Work out the finished part from the listing and answer in its coordinate system (mm). A direction names the side the tool comes from. Coordinates: 2 decimals unless noted, no trailing zeros. Loops run counter-clockwise (first coordinate to the right, second up) from the corner with the lowest first, then second, coordinate; pieces in that order, holes last. Notation, with made-up numbers: (43.25, 26.5) - (51.25, 26.5) arc R9 cw to (51.25, 42.5) - close; hole circle Ø7 at (80, 82). An arc over 180 degrees is marked (long way). Write each question's results on one line, items separated by ' | '. Start each with the question number.
Item 1: Section A-A, the plane x = -9.75 is taken. Write down the section's boundary in (y, z), plus the area to 3 significant figures.
Item 2: Section C-C, the plane y = 6.75 is taken. Write down the section's boundary in (x, z), plus the area to 3 significant figures.
Item 3: Section B-B, the plane x = 0 is taken. Write down the section's boundary in (y, z) (3 decimals).
Item 4: Each of these flat-tipped pins is pushed along its axis until it touches: pin 1 Ø2.5 at (y, z) = (-4.5, -0.5) entering from -X; pin 2 Ø3 at (x, y) = (2, 9) entering from -Z; pin 3 Ø10 at (x, y) = (6.5, 6) entering from -Z; pin 4 Ø0.6 at (y, z) = (-2, -1.5) entering from +X (3 decimals). Where does it stop, or does it pass through?
Item 5: A tool of negligible diameter and unlimited length cuts with its end or side. For faces 4 (the face through (0, -6.64, -1)), 5 (the face through (-3.7, -3.4, -2.25)), 6 (the face through (11.86, 11.32, 0.49)), 7 (the face through (4.215, -2, -1)), 8 (the face through (0, -2, -4.5)), from which of +Z, -Z, +X, -X, +Y, -Y can it reach the whole face along a straight path? Write none if from no direction.
Item 6: For a pull along X with two mould halves and no side action, classify faces 1 (the face through (-1, 0, -4)), 2 (the face through (0, 0, 1)), 3 (the face through (-12.5, 0.1, 0.5)) as +X half, -X half, draft (parallel to the pull), parting line (faces both ways), or undercut.
Item 7: Section D-D, the plane z = -1.3 is taken. Write down the section's boundary in (x, y) (3 decimals), plus the area to 3 significant figures.
Item 8: Consider probe 1 along Y at (x, z) = (0, -4.2) (3 decimals); probe 2 along Z at (x, y) = (8.5, 5.75); probe 3 along X at (y, z) = (-2, -0.6) (3 decimals). Determine where each line is inside the solid, lowest interval first. Write a range as [from, to].
from build123d import *

# Parameters (mm, degrees)
F0_R     = 1.075
F1_DEPTH = 1
F2_W     = 8.43
F2_H     = 8.43
F3_DEPTH = 2.25
F4_R     = 3.65
F5_DEPTH = 2.25
F7_R     = 2.9
F7_R_2   = 2.15
F8_DEPTH = 0.5
F9_R     = 0.1


with BuildPart() as f1:
    # F0 (on Top) → F1 (new body)
    with BuildSketch(Plane.XY):
        with BuildLine():
            ThreePointArc((12.5, 9.75), (11.84099, 11.34099), (10.25, 12))
            Line((10.25, 12), (-10.25, 12))
            ThreePointArc((-10.25, 12), (-11.84099, 11.34099), (-12.5, 9.75))
            Line((-12.5, 9.75), (-12.5, -9.75))
            ThreePointArc((-12.5, -9.75), (-11.84099, -11.34099), (-10.25, -12))
            Line((-10.25, -12), (10.25, -12))
            ThreePointArc((10.25, -12), (11.84099, -11.34099), (12.5, -9.75))
            Line((12.5, -9.75), (12.5, 9.75))
        make_face()
        with Locations((-10.525, -2.575)):
            Circle(F0_R, mode=Mode.SUBTRACT)
        with Locations((10.525, -2.575)):
            Circle(F0_R, mode=Mode.SUBTRACT)
        with Locations((-10.525, 10.025)):
            Circle(F0_R, mode=Mode.SUBTRACT)
        with Locations((10.525, 10.025)):
            Circle(F0_R, mode=Mode.SUBTRACT)
    extrude(amount=F1_DEPTH)

    # F2 (on face) → F3 (join)
    with BuildSketch(Plane(origin=(0, 0, 0), x_dir=(1, 0, 0), z_dir=(0, 0, -1))):
        with Locations((0, 2.425)):
            Rectangle(F2_W, F2_H)
    extrude(amount=F3_DEPTH)

    # F4 (on face) → F5 (join)
    with BuildSketch(Plane(origin=(0, 0, -2.25), x_dir=(1, 0, 0), z_dir=(0, 0, -1))):
        with Locations((0, 2.425)):
            Circle(F4_R)
    extrude(amount=F5_DEPTH)

    # F7 (on face) → F8 (cut)
    with BuildSketch(Plane(origin=(0, 0, -4.5), x_dir=(1, 0, 0), z_dir=(0, 0, -1))):
        with Locations((0, 2.425)):
            Circle(F7_R)
        with Locations((0, 2.425)):
            Circle(F7_R_2, mode=Mode.SUBTRACT)
    extrude(amount=-F8_DEPTH, mode=Mode.SUBTRACT)

    # F9
    f9_edges = [f1.edges().sort_by_distance(p)[0] for p in [
        (-2.9, -2.425, -4),
        (-2.9, -2.425, -4.5),
        (0, 1.79, -2.25),
        (4.215, -2.425, -2.25),
        (0, -6.64, -2.25),
        (-4.215, -2.425, -2.25),
    ]]
    fillet(f9_edges, radius=F9_R)


solid = f1.part
Answer key:
1) outline: (-12, 0) - (-3.32, 0) - (-3.32, 1) - (-12, 1) - close; (-1.83, 0) - (9.28, 0) - (9.28, 1) - (-1.83, 1) - close; (10.77, 0) - (12, 0) - (12, 1) - (10.77, 1) - close | area: 21.0 mm^2
2) outline: (-12.5, 0) - (12.5, 0) - (12.5, 1) - (-12.5, 1) - close | area: 25.0 mm^2
3) outline: (-12, 0) - (-6.64, 0) - (-6.64, -2.15) arc R0.1 ccw to (-6.54, -2.25) - (-6.075, -2.25) - (-6.075, -4.5) - (-5.425, -4.5) arc R0.1 ccw to (-5.325, -4.4) - (-5.325, -4.1) arc R0.1 cw to (-5.225, -4) - (-4.575, -4) - (-4.575, -4.5) - (-0.275, -4.5) - (-0.275, -4) - (0.375, -4) arc R0.1 cw to (0.475, -4.1) - (0.475, -4.4) arc R0.1 ccw to (0.575, -4.5) - (1.225, -4.5) - (1.225, -2.25) - (1.69, -2.25) arc R0.1 ccw to (1.79, -2.15) - (1.79, 0) - (12, 0) - (12, 1) - (-12, 1) - close
4) pin 1: stops at x = -12.5 | pin 2: stops at z = 0 | pin 3: stops at z = -2.25 | pin 4: stops at x = 4.215
5) face 4: -Z, +X, -X, -Y | face 5: -Z | face 6: +Z, -Z, +X, +Y | face 7: -Z, +X, +Y, -Y | face 8: -Z, +X, -X, +Y, -Y
6) face 1: undercut | face 2: draft | face 3: -X half
7) outline: (-4.215, -6.64) - (4.215, -6.64) - (4.215, 1.79) - (-4.215, 1.79) - close | area: 71.1 mm^2
8) probe 1: y = [-6.075, -5.325], [-4.575, -0.275], [0.475, 1.225] | probe 2: z = [0, 1] | probe 3: x = [-4.215, 4.215]
